from build123d import *

# Parameters (mm, degrees)
SKETCH1_W               = 60
SKETCH1_H               = 78
SKETCH1_W_2             = 54
SKETCH1_H_2             = 72
EXTRUDE_THIN1_DEPTH     = 3
EXTRUDE_THIN2_DEPTH     = 3
BOSS_EXTRUDE1_DEPTH     = 7
SKETCH5_W               = 9
SKETCH5_H               = 3
BOSS_EXTRUDE2_DEPTH     = 10
SKETCH5_W_2             = 14
BOSS_EXTRUDE2_2_DEPTH   = 10
SKETCH6_W               = 3
SKETCH6_H               = 3
BOSS_EXTRUDE3_DEPTH     = 3
CUT_EXTRUDE1_DEPTH      = 95.731198662
SKETCH9_W               = 54
SKETCH9_H               = 3
BOSS_EXTRUDE4_DEPTH     = 3
FILLET1_R               = 7
FILLET2_R               = 10
CUT_EXTRUDE2_REACH      = 92.526
CUT_EXTRUDE3_DEPTH      = 97.922649572
CUT_EXTRUDE3_DEPTH_BACK = 97.922649572
SKETCH11_W              = 3
SKETCH11_H              = 3
FILLET3_R               = 1
CUT_EXTRUDE4_DEPTH      = 95.731198812
FILLET4_R               = 12
SKETCH14_W              = 3
SKETCH14_H              = 3
BOSS_EXTRUDE5_DEPTH     = 3


# Read off the part's stored shape, not the designer's step: Extrude-Thin2
# Some blends are built 0.0001 mm under size
with BuildPart() as part:
    # Sketch1 → Extrude-Thin1 (new body)
    with BuildSketch(Plane(origin=(0, 0, 0), x_dir=(1, 0, 0), z_dir=(0, 1, 0))):
        with Locations((27, 36)):
            Rectangle(SKETCH1_W, SKETCH1_H)
        with Locations((27, 36)):
            Rectangle(SKETCH1_W_2, SKETCH1_H_2, mode=Mode.SUBTRACT)
    extrude(amount=EXTRUDE_THIN1_DEPTH)

    # Extrude-Thin2 outline → Extrude-Thin2 (add)
    with BuildSketch(Plane(origin=(0, 0, 0), x_dir=(1, 0, 0), z_dir=(0, 1, 0))):
        Polygon((0, 69.878679656), (7.232233047, 62.646446609), (0, 55.414213562), (0, 51.878679656), (6.878679656, 45), (0, 38.121320344), (0, 34.585786438), (7.232233047, 27.353553391), (0, 20.121320344), (0, 15.878679656), (7.232233047, 8.646446609), (0, 1.414213562), (0, 0), (2.121320344, 0), (9, 6.878679656), (15.878679656, 0), (20.121320344, 0), (27.353553391, 7.232233047), (34.585786438, 0), (38.121320344, 0), (45, 6.878679656), (51.878679656, 0), (54, 0), (54, 1.414213562), (46.767766953, 8.646446609), (54, 15.878679656), (54, 19.414213562), (46.767766953, 26.646446609), (54, 33.878679656), (54, 37.414213562), (46.767766953, 44.646446609), (54, 51.878679656), (54, 55.414213562), (46.414213562, 63), (54, 70.585786438), (54, 72), (51.878679656, 72), (44.646446609, 64.767766953), (37.414213562, 72), (33.878679656, 72), (26.646446609, 64.767766953), (19.414213562, 72), (16.585786438, 72), (9, 64.414213562), (1.414213562, 72), (0, 72), align=None)
        Polygon((10.767766953, 8.646446609), (18.353553391, 16.232233047), (25.585786438, 9), (18, 1.414213562), align=None, mode=Mode.SUBTRACT)
        Polygon((9, 10.414213562), (1.414213562, 18), (9, 25.585786438), (16.585786438, 18), align=None, mode=Mode.SUBTRACT)
        Polygon((18.353553391, 19.767766953), (10.767766953, 27.353553391), (17.646446609, 34.232233047), (25.232233047, 26.646446609), align=None, mode=Mode.SUBTRACT)
        Polygon((26.646446609, 43.232233047), (34.232233047, 35.646446609), (27, 28.414213562), (19.414213562, 36), align=None, mode=Mode.SUBTRACT)
        Polygon((29.121320344, 9), (36, 15.878679656), (43.232233047, 8.646446609), (36.353553391, 1.767766953), align=None, mode=Mode.SUBTRACT)
        Polygon((20.121320344, 18), (27, 24.878679656), (34.232233047, 17.646446609), (27.353553391, 10.767766953), align=None, mode=Mode.SUBTRACT)
        Polygon((45, 24.878679656), (52.232233047, 17.646446609), (45, 10.414213562), (37.767766953, 17.646446609), align=None, mode=Mode.SUBTRACT)
        Polygon((36, 33.878679656), (43.232233047, 26.646446609), (36, 19.414213562), (28.767766953, 26.646446609), align=None, mode=Mode.SUBTRACT)
        Polygon((52.232233047, 35.646446609), (45, 28.414213562), (37.767766953, 35.646446609), (45, 42.878679656), align=None, mode=Mode.SUBTRACT)
        Polygon((15.878679656, 36), (9, 29.121320344), (1.767766953, 36.353553391), (8.646446609, 43.232233047), align=None, mode=Mode.SUBTRACT)
        Polygon((9, 60.878679656), (15.878679656, 54), (8.646446609, 46.767766953), (1.767766953, 53.646446609), align=None, mode=Mode.SUBTRACT)
        Polygon((17.646446609, 52.232233047), (24.878679656, 45), (17.646446609, 37.767766953), (10.414213562, 45), align=None, mode=Mode.SUBTRACT)
        Polygon((24.878679656, 63), (17.646446609, 55.767766953), (10.767766953, 62.646446609), (18, 69.878679656), align=None, mode=Mode.SUBTRACT)
        Polygon((33.878679656, 54), (26.646446609, 46.767766953), (19.414213562, 54), (26.646446609, 61.232233047), align=None, mode=Mode.SUBTRACT)
        Polygon((43.232233047, 44.646446609), (36, 37.414213562), (28.414213562, 45), (35.646446609, 52.232233047), align=None, mode=Mode.SUBTRACT)
        Polygon((45, 46.414213562), (37.414213562, 54), (44.646446609, 61.232233047), (52.232233047, 53.646446609), align=None, mode=Mode.SUBTRACT)
        Polygon((42.878679656, 63), (35.646446609, 55.767766953), (28.414213562, 63), (35.646446609, 70.232233047), align=None, mode=Mode.SUBTRACT)
    extrude(amount=EXTRUDE_THIN2_DEPTH)

    # Sketch4 → Boss-Extrude1 (add)
    with BuildSketch(Plane(origin=(0, 3, 0), x_dir=(1, 0, 0), z_dir=(0, 1, 0))):
        Polygon((0, 0), (0, 72), (0, 75), (-3, 75), (-3, -3), (57, -3), (57, 75), (54, 75), (54, 72), (54, 0), align=None)
    extrude(amount=BOSS_EXTRUDE1_DEPTH)

    # Sketch6 → Boss-Extrude3 (add)
    with BuildSketch(Plane.XZ):
        with Locations((-1.5, 1.5)):
            Rectangle(SKETCH6_W, SKETCH6_H)
    extrude(amount=BOSS_EXTRUDE3_DEPTH)

    # Sketch7 → Cut-Extrude1 (cut, through all)
    with BuildSketch(Plane(origin=(0, 3, 0), x_dir=(1, 0, 0), z_dir=(0, 1, 0))):
        Polygon((33.878679656, 72), (36.878679656, 75), (16.414213562, 75), (0, 75), (0, 73.5), (1.414213562, 72), (17.646446609, 55.767766953), (26.646446609, 64.767766953), align=None)
    extrude(amount=-CUT_EXTRUDE1_DEPTH, mode=Mode.SUBTRACT)



with BuildPart() as body_2:
    # Sketch5 → Boss-Extrude2 (new body)
    with BuildSketch(Plane(origin=(0, 0, 0), x_dir=(-1, 0, 0), z_dir=(0, 0, -1))):
        with Locations((-41.5, 11.5)):
            Rectangle(SKETCH5_W, SKETCH5_H)
    extrude(amount=BOSS_EXTRUDE2_DEPTH)


with BuildPart() as body_3:
    # Sketch5 → Boss-Extrude2 2 (new body)
    with BuildSketch(Plane(origin=(0, 0, 0), x_dir=(-1, 0, 0), z_dir=(0, 0, -1))):
        with Locations((-15, 11.5)):
            Rectangle(SKETCH5_W_2, SKETCH5_H)
    extrude(amount=BOSS_EXTRUDE2_2_DEPTH)


with BuildPart() as part_1:
    add(part.part)

    add(body_2.part)  # Boss-Extrude4 merges body 2

    add(body_3.part)  # Boss-Extrude4 merges body 3
    # Sketch9 → Boss-Extrude4 (add)
    with BuildSketch(Plane.XY):
        with Locations((27, 11.5)):
            Rectangle(SKETCH9_W, SKETCH9_H)
    extrude(amount=BOSS_EXTRUDE4_DEPTH)

    # Fillet1
    fillet1_edges = [part_1.edges().sort_by_distance(p)[0] for p in [
        (41.5, 10, 0),
        (15, 10, 0),
    ]]
    fillet(fillet1_edges, radius=FILLET1_R - 0.0001)  # a hair under: the kernel refuses the full size

    # Fillet2
    # the kernel refuses this fillet: 10 mm, written as the material it takes off along each edge
    with BuildSketch(Plane(origin=(79, 13, 3), x_dir=(0, -1, 0), z_dir=(-1, 0, 0))) as fillet2_piece_1:
        with BuildLine():
            CenterArc((FILLET2_R, -FILLET2_R), FILLET2_R, 90, 90)
            Line((0, -FILLET2_R), (0, 0))
            Line((0, 0), (FILLET2_R, 0))
        make_face()
    extrude(amount=104, mode=Mode.SUBTRACT)

    # Sketch10 → Cut-Extrude2 (cut, up to next)
    with BuildSketch(Plane.ZY.offset(-8), mode=Mode.PRIVATE) as cut_extrude2_sk1:
        with BuildLine():
            ThreePointArc((-7, 10), (-8.5, 11.5), (-7, 13))
            Line((-7, 13), (-10, 13))
            Line((-10, 13), (-10, 10))
            Line((-10, 10), (-7, 10))
        make_face()
    cut_extrude2_tool1 = extrude(cut_extrude2_sk1.sketch, amount=-CUT_EXTRUDE2_REACH, mode=Mode.PRIVATE) & part_1.part
    add(cut_extrude2_tool1.solids().sort_by_distance((8, 11.5, -9.058288))[0], mode=Mode.SUBTRACT)
    add(cut_extrude2_tool1.solids().sort_by_distance((8, 11.5, -9.058288))[1], mode=Mode.SUBTRACT)

    # Sketch11 → Cut-Extrude3 (cut, two sides: drawn at the far end of the back side and taken through both)
    with BuildSketch(Plane.ZY.offset(3).offset(-CUT_EXTRUDE3_DEPTH_BACK)):
        with Locations((1.5, -1.5)):
            Rectangle(SKETCH11_W, SKETCH11_H)
    extrude(amount=CUT_EXTRUDE3_DEPTH + CUT_EXTRUDE3_DEPTH_BACK, mode=Mode.SUBTRACT)

    # Fillet3
    fillet3_edges = [part_1.edges().sort_by_distance(p)[0] for p in [
        (57, 10, -37.429285786),
        (-3, 10, -37.429285786),
        (-3, 5, -75),
        (57, 5, -75),
    ]]
    fillet(fillet3_edges, radius=FILLET3_R)

    # Sketch12 → Cut-Extrude4 (cut, through all)
    with BuildSketch(Plane(origin=(0, 3, 0), x_dir=(1, 0, 0), z_dir=(0, 1, 0))):
        Polygon((17.646446609, 55.767766953), (26.646446609, 46.767766953), (54, 74.121320344), (54, 75), (17.646446609, 75), align=None)
    extrude(amount=-CUT_EXTRUDE4_DEPTH, mode=Mode.SUBTRACT)

    # Fillet4
    fillet4_edges = [part_1.edges().sort_by_distance(p)[0] for p in [
        (26.646446609, 1.5, -46.767766953),
    ]]
    fillet(fillet4_edges, radius=FILLET4_R)

    # Sketch14 → Boss-Extrude5 (add)
    with BuildSketch(Plane.XZ):
        with Locations((-1.5, 1.5)):
            Rectangle(SKETCH14_W, SKETCH14_H)
    extrude(amount=BOSS_EXTRUDE5_DEPTH)


solid = part_1.part
Can you work these out from the model? Positions are in its coordinate system, mm. A direction names the side the tool comes from. Give positions to 0.01 mm unless a question says otherwise; leave off trailing zeros. Loops run counter-clockwise (first coordinate to the right, second up) from the corner with the lowest first, then second, coordinate; pieces in that order, holes last. Notation, with made-up numbers: (58, 15) -> (81, 15) arc R25 cw to (81, 34) -> close; hole circle Ø9 at (69.5, 82.25). An arc over 180 degrees is marked (long way). Write item = value, one per line.
1) Will these pins go through, and if not, where does the flat tip stop? pin 1 (16 mm diameter, centred on x = 22.5, z = -50, fed in from +Y); pin 2 (3 mm diameter, centred on x = 27, y = 5.5, fed in from +Z); pin 3 (0.9 mm diameter, centred on y = -1.5, z = 1, fed in from +X).
Check result:
pin_1 = 3
pin_2 = 2.95
pin_3 = 0
2) I need wall thicknesses on L1, parallel to X at y = 3.25, z = -42.5; L2, parallel to Z at x = 28, y = 1; L3, parallel to X at y = 0.5, z = -8. Which ranges of each line are inside material? Lowest first, please. Write a range as from..to.
Check result:
L1 = -3..0, 54..57
L2 = -51.81..-41.88, -29.41..-23.88, -11.41..-6.59, 0..3
L3 = -3..0, 6.59..11.41, 24.59..30.12, 42.59..47.41, 54..57
3) Suppose I cut it at D-D on y = 5. Write out the boundary of the cut face in (x, z), then the cut area to 3 significant figures.
Check result:
outline = (-3, -74) arc R1 ccw to (-2, -75) -> (0, -75) -> (0, 0) -> (8, 0) -> (8, -0.29) -> (22, -0.29) -> (22, 0) -> (37, 0) -> (37, -0.29) -> (46, -0.29) -> (46, 0) -> (54, 0) -> (54, -75) -> (56, -75) arc R1 ccw to (57, -74) -> (57, 2.8) -> (-3, 2.8) -> close
area = 624 mm2
4) Suppose I cut it at B-B on y = 11.5. Write out the boundary of the cut face in (x, z).
Check result:
outline = (8, -8.5) -> (22, -8.5) -> (22, -1.73) -> (8, -1.73) -> close; (37, -8.5) -> (46, -8.5) -> (46, -1.73) -> (37, -1.73) -> close
5) Thinking about a two-plate mould opening in Z: for faces 1 (the flat face through (57, 4, -35)), 2 (the flat face through (55, 5, -75)), 3 (the flat face through (48.57, 1.48, -21.31)), which applies, released by +Z, released by -Z, zero draft, split by the parting line, or undercut?
Check result:
face_1 = zero draft
face_2 = released by -Z
face_3 = undercut
6) Suppose I cut it at A-A on z = -49. Give the number of separate pieces and of enclosed holes in the cut face, then the cut area to 3 significant figures.
Check result:
separate_pieces = 7
enclosed_holes = 0
area = 137 mm2
7) For faces 4 (the cylindrical face through (14.9, 7.9, -2)), 5 (the flat face through (0, 5, -37)), 6 (the flat face through (0, -1, 1)), 7 (the flat face through (9.905, 1.479, -63.509)), which set-ups out of +Z, -Z, +X, -X, +Y, -Y let a thin tool reach every point of the face, with its end or its side?
Check result:
face_4 = -Z
face_5 = +Y
face_6 = +Z, -Z, +X, -Y
face_7 = -Z, +Y, -Y
